from build123d import *

# Parameters (mm, degrees)
BOSS_EXTRUDE2_DEPTH      = 1.5
SKETCH2_R                = 2.5
BOSS_EXTRUDE3_DEPTH      = 1.5
FILLET2_R                = 1
SKETCH3_R                = 2
BOSS_EXTRUDE4_DEPTH      = 10
BOSS_EXTRUDE5_DEPTH      = 5
BOSS_EXTRUDE5_DEPTH_BACK = 11
SKETCH6_R                = 2.5
SKETCH7_R                = 2.5
BOSS_EXTRUDE6_DEPTH      = 11
SKETCH8_R                = 2.5
BOSS_EXTRUDE7_DEPTH      = 8


with BuildPart() as part:
    # Sketch1 → Boss-Extrude2 (new body)
    with BuildSketch(Plane.XY):
        with BuildLine():
            Line((-35, 5), (25, 5))
            Line((25, 5), (25, -5))
            Line((25, -5), (-35, -5))
            ThreePointArc((-35, -5), (-30, 0), (-35, 5))
        make_face()
    boss_extrude2 = extrude(amount=BOSS_EXTRUDE2_DEPTH)

    # Sketch2 → Boss-Extrude3 (add)
    with BuildSketch(Plane.XY.offset(1.5)):
        with Locations(Location((20, 0, 0), (0, 0, 180))):
            Circle(SKETCH2_R)
        with BuildLine():
            Line((-32, -9.19371522), (-32, -7))
            ThreePointArc((-32, -7), (-29.141428429, 0), (-32, 7))
            Line((-32, 7), (-32, 9.19371522))
            ThreePointArc((-32, 9.19371522), (-30.857040195, 11.549856497), (-28.299065524, 12.110681257))
            Line((-28.299065524, 12.110681257), (-8.247663809, 7.292415092))
            ThreePointArc((-8.247663809, 7.292415092), (-2.5, 0), (-8.247663809, -7.292415092))
            Line((-8.247663809, -7.292415092), (-28.299065524, -12.110681257))
            ThreePointArc((-28.299065524, -12.110681257), (-30.857040195, -11.549856497), (-32, -9.19371522))
        make_face()
    boss_extrude3 = extrude(amount=BOSS_EXTRUDE3_DEPTH)

    # Mirror1: Boss-Extrude2, Boss-Extrude3 across plane
    add(boss_extrude2.mirror(Plane(origin=(-35, 0, 0), x_dir=(1, 0, 0), z_dir=(0, 0, -1))))
    add(boss_extrude3.mirror(Plane(origin=(-35, 0, 0), x_dir=(1, 0, 0), z_dir=(0, 0, -1))))

    # Fillet2
    fillet2_edges = [part.edges().sort_by_distance(p)[0] for p in [
        (-35, -5, 0),
        (-35, 5, 0),
    ]]
    fillet(fillet2_edges, radius=FILLET2_R)

    # Sketch3 → Boss-Extrude4 (add)
    with BuildSketch(Plane.XY.offset(3)):
        with Locations(Location((-7, 0, 0), (0, 0, 180))):
            Circle(SKETCH3_R)
    extrude(amount=BOSS_EXTRUDE4_DEPTH)

    # Sketch6 → Boss-Extrude5 (add, two sides: drawn at the far end of the back side and taken through both)
    with BuildSketch(Plane.XY.offset(3).offset(-BOSS_EXTRUDE5_DEPTH_BACK)):
        with Locations(Location((20, 0, 0), (0, 0, 180))):
            Circle(SKETCH6_R)
    extrude(amount=BOSS_EXTRUDE5_DEPTH + BOSS_EXTRUDE5_DEPTH_BACK)

    # Sketch7 → Boss-Extrude6 (add)
    with BuildSketch(Plane(origin=(0, 0, -3), x_dir=(-1, 0, 0), z_dir=(0, 0, -1))):
        with Locations(Location((15, 0, 0), (0, 0, 180))):
            Circle(SKETCH7_R)
    extrude(amount=BOSS_EXTRUDE6_DEPTH)

    # Sketch8 → Boss-Extrude7 (add)
    with BuildSketch(Plane(origin=(0, 0, -1.5), x_dir=(-1, 0, 0), z_dir=(0, 0, -1))):
        with Locations(Location((-1, 0, 0), (0, 0, 180))):
            Circle(SKETCH8_R)
    extrude(amount=BOSS_EXTRUDE7_DEPTH)


solid = part.part
Design review of the part built by this model. Coordinates are the model's own, in mm. A direction names the side the tool comes from. Round coordinates to 2 decimals unless told otherwise and drop trailing zeros. Write each loop counter-clockwise with the first axis right and the second up, starting at its lowest first coordinate (ties: lowest second). Pieces come first, ordered by that corner, then holes. Notation, with made-up numbers: (-0.75, 6.5) -> (6.25, 6.5) arc R32 ccw to (6.25, 34.5) -> close; hole circle Ø4 at (24, -21.5). An arc over 180 degrees is marked (long way). One line per item, written item: value. Start each with the question number.
Q1. Insertion check: P1, Ø5, axis at x = -23.5, y = -6, coming from the +Z side; P2, Ø0.7, axis at x = -30, y = 2, coming from the +Z side; P3, Ø4, axis at x = 20.5, y = 1, coming from the -Z side. Each pin has a flat end and moves straight along its axis. Give the tip position at first contact, or say it passes through.
Q2. To check wall thickness, follow probe 1 along Z at (x, y) = (7.5, 0.75); probe 2 along Z at (x, y) = (0, 2.25); probe 3 along X at (y, z) = (1.75, 5.75). State the ranges of each line that lie inside material, in increasing order.
Q3. Add section A-A (x = 20). Give the boundary of the cut face in (y, z).
Q4. Tool access review of faces 5 (the face through (-2, -5, 0)), 6 (the face through (-21, 8, 1.5)), 7 (the face through (3.385, -0.751, -5.444)): name each direction out of +Z, -Z, +X, -X, +Y, -Y from which nothing blocks a thin tool from reaching the whole face with its end or side.
Q5. Add section D-D (x = 1). Give the boundary of the cut face in (y, z), then the cut area to 3 significant figures.
Q6. Add section B-B (z = -12). Give the boundary of the cut face in (x, y), then the cut area to 3 significant figures.
Q7. The part is to be moulded in two halves that separate along X. For faces 1 (the face through (-18.414, 9.735, -2.24)), 2 (the face through (-29.8, 0.1, 1.5)), 3 (the face through (-32, 8, 2)), 4 (the face through (22.5, -0.1, -4.8)), say which applies: pulls with the +X half, pulls with the -X half, needs draft (parallel to the pull), parting line crosses it, or undercut.
Response:
1. P1: stops at z = 3
1. P2: stops at z = 1.5
1. P3: stops at z = -8
2. probe 1: z = -1.5 to 1.5
2. probe 2: z = -9.5 to 1.5
2. probe 3: x = -7.97 to -6.03, 18.21 to 21.79
3. outline: (-5, -1.5) -> (-2.5, -1.5) -> (-2.5, -8) -> (2.5, -8) -> (2.5, -1.5) -> (5, -1.5) -> (5, 1.5) -> (2.5, 1.5) -> (2.5, 8) -> (-2.5, 8) -> (-2.5, 1.5) -> (-5, 1.5) -> close
4. face 5: +X, -X, -Y
4. face 6: +X, -X, +Y
4. face 7: -Z
5. outline: (-5, -1.5) -> (-2.5, -1.5) -> (-2.5, -9.5) -> (2.5, -9.5) -> (2.5, -1.5) -> (5, -1.5) -> (5, 1.5) -> (-5, 1.5) -> close
5. area: 70.0 mm^2
6. outline: circle Ø5 at (-15, 0)
6. area: 19.6 mm^2
7. face 1: pulls with the +X half
7. face 2: needs draft
7. face 3: pulls with the -X half
7. face 4: undercut
